Geometry: see drawing. Coordinates: mm, zero at the bounding-box minimum. A direction names the side the tool comes from. Coordinates: 2 decimals unless noted, no trailing zeros. Write each loop counter-clockwise with the first axis right and the second up, starting at its lowest first coordinate (ties: lowest second). Pieces come first, ordered by that corner, then holes. Notation, with made-up numbers: (20.25, 80) - (79.25, 80) arc R23 ccw to (79.25, 95) - close; hole circle Ø2 at (15, 17.5). An arc over 180 degrees is marked (long way). Use a Markdown table: item, result. Add a question column.
Q1. Section query B-B (y = 10.5). Return the cut outline in (x, z), then the cut area to 3 significant figures.
Q2. Section query A-A (z = 22.5). Return the cut outline in (x, y).
Q3. Material intervals for probe 1 along Z at (x, y) = (0.6, 9.5); probe 2 along Z at (x, y) = (13, 0.5); probe 3 along X at (y, z) = (0.6, 10), sorted ascending. Write a range as from..to.
Q4. Section query C-C (x = 3.25). Return the cut outline in (y, z).
Q5. Pin query (flat end, axial travel): P1, Ø1.5, axis at x = 11, z = 13.5, coming from the +Y side; P2, Ø5.5, axis at y = 12, z = 10.5, coming from the +X side. Return the tip coordinate at first contact, or that it passes through.
Q6. Set-up query: the marked faces 1 and 2. Return all of +Z, -Z, +X, -X, +Y, -Y with unobstructed straight access to the full face (end or side cutting, diameter ignored); none if empty.
Q7. Section query D-D (z = 6.75). Return the cut outline in (x, y), then the cut area to 3 significant figures.
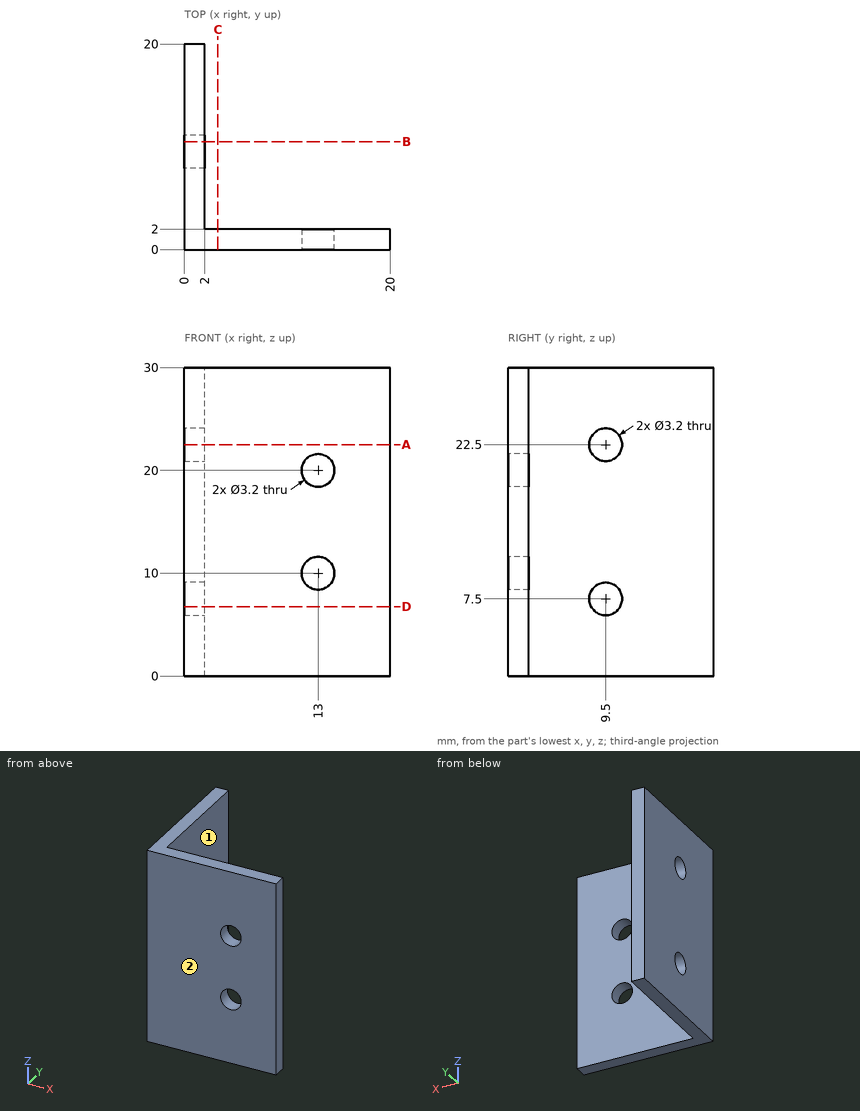
Values follow:
| question | item | result |
|---|---|---|
| 1 | outline | (0, 0) - (2, 0) - (2, 6.25) - (0, 6.25) - close; (0, 8.75) - (2, 8.75) - (2, 21.25) - (0, 21.25) - close; (0, 23.75) - (2, 23.75) - (2, 30) - (0, 30) - close |
| 1 | area | 50.0 mm2 |
| 2 | outline | (0, 0) - (20, 0) - (20, 2) - (2, 2) - (2, 7.9) - (0, 7.9) - close; (0, 11.1) - (2, 11.1) - (2, 20) - (0, 20) - close |
| 3 | probe 1 | 0..5.9, 9.1..20.9, 24.1..30 |
| 3 | probe 2 | 0..8.4, 11.6..18.4, 21.6..30 |
| 3 | probe 3 | 0..11.4, 14.6..20 |
| 4 | outline | (0, 0) - (2, 0) - (2, 30) - (0, 30) - close |
| 5 | P1 | y = 2 |
| 5 | P2 | x = 2 |
| 6 | face 1 | +Z, -Z, +X, +Y |
| 6 | face 2 | +Z, -Z, +X, -X, -Y |
| 7 | outline | (0, 0) - (20, 0) - (20, 2) - (2, 2) - (2, 8.09) - (0, 8.09) - close; (0, 10.91) - (2, 10.91) - (2, 20) - (0, 20) - close |
| 7 | area | 70.3 mm2 |
